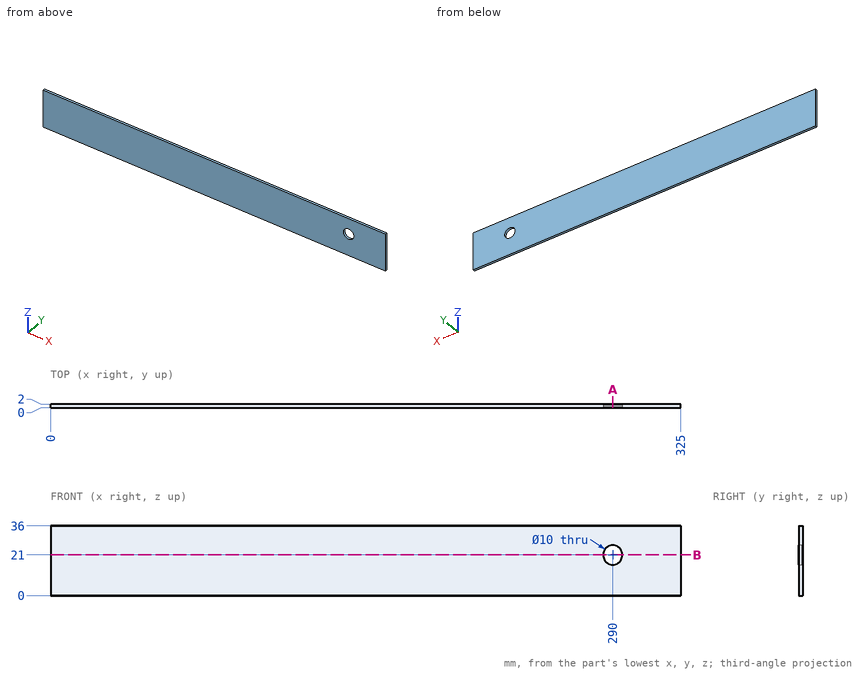
The drawing under review shows one solid part. Ordinate dimensions are in mm from its lowest x, y, z. Round coordinates to 2 decimals unless told otherwise and drop trailing zeros. Write each loop counter-clockwise with the first axis right and the second up, starting at its lowest first coordinate (ties: lowest second). Pieces come first, ordered by that corner, then holes. Notation, with made-up numbers: (14, 40.5) - (73, 40.5) arc R13 ccw to (73, 62.5) - close; hole circle Ø1 at (60, -38.5). An arc over 180 degrees is marked (long way). Put each result on its own line as item: value.
Q1. Insertion check: pin 1 Ø6 at (x, z) = (290, 21) entering from +Y. The pin has a flat end and moves straight along its axis. Give the tip position at first contact, or say it passes through.
Solved:
pin 1: passes through
Q2. We need section A-A (x = 290). Give the boundary of the cut face in (y, z), and give its area (3 significant figures).
Solved:
outline: (0, 0) - (2, 0) - (2, 16) - (0, 16) - close; (0, 26) - (2, 26) - (2, 36) - (0, 36) - close
area: 52.0 mm2
Q3. We need section B-B (z = 21). Give the boundary of the cut face in (x, y).
Solved:
outline: (0, 0) - (285, 0) - (285, 2) - (0, 2) - close; (295, 0) - (325, 0) - (325, 2) - (295, 2) - close
Q4. Wall thickness on probe 1 along Z at (x, y) = (290, 1.5); probe 2 along X at (y, z) = (1.3, 21); probe 3 along X at (y, z) = (1.4, 19): over which ranges is each line inside the solid? List them lowest first.
Solved:
probe 1: z = 0 to 16, 26 to 36
probe 2: x = 0 to 285, 295 to 325
probe 3: x = 0 to 285.42, 294.58 to 325
